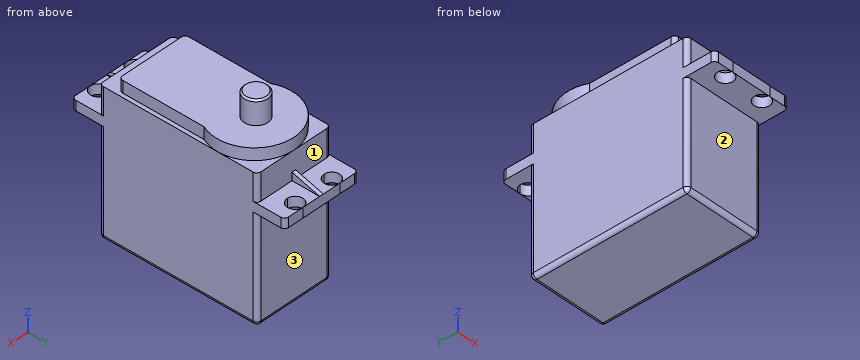
```python
from build123d import *

# Parameters (mm, degrees)
SKETCH_W        = 54
SKETCH_H        = 36
PAD_DEPTH       = 20
SKETCH001_W     = 7
SKETCH001_H     = 26.6
SKETCH001_H_2   = 6.9
POCKET_DEPTH    = 20.001
PAD001_DEPTH    = 3
SKETCH003_R     = 3
PAD002_DEPTH    = 45
SKETCH004_R     = 2
POCKET001_DEPTH = 2.5
PAD003_START    = -9.5
PAD003_DEPTH    = 1
CHAMFER_SIZE    = 0.4
FILLET_R        = 1
FILLET001_R     = 1
FILLET002_R     = 1


with BuildPart() as part:
    # Sketch → Pad (new body)
    with BuildSketch(Plane.YZ):
        with Locations((27, 18)):
            Rectangle(SKETCH_W, SKETCH_H)
    extrude(amount=PAD_DEPTH)

    # Sketch001 (on DatumPlane) → Pocket (cut, through all)
    with BuildSketch(Plane.YZ.offset(20)):
        with Locations((3.5, 13.3)):
            Rectangle(SKETCH001_W, SKETCH001_H)
        with Locations((50.5, 13.3)):
            Rectangle(SKETCH001_W, SKETCH001_H)
        with Locations((3.5, 32.55)):
            Rectangle(SKETCH001_W, SKETCH001_H_2)
        with Locations((50.5, 32.55)):
            Rectangle(SKETCH001_W, SKETCH001_H_2)
    extrude(amount=-POCKET_DEPTH, mode=Mode.SUBTRACT)

    # Sketch002 (on DatumPlane) → Pad001 (join)
    with BuildSketch(Plane(origin=(0, 0, 36), x_dir=(0, -1, 0), z_dir=(0, 0, 1))):
        with BuildLine():
            Line((-11, 19), (-32.641101, 19))
            ThreePointArc((-32.641101, 19), (-47, 10), (-32.641101, 1))
            Line((-32.641101, 1), (-11, 1))
            Line((-11, 1), (-11, 19))
        make_face()
    extrude(amount=PAD001_DEPTH)

    # Sketch003 → Pad002 (join)
    with BuildSketch(Plane.XY):
        with Locations((10, 37.4)):
            Circle(SKETCH003_R)
    extrude(amount=PAD002_DEPTH)

    # Sketch004 (on Face7 of Pad002) → Pocket001 (cut)
    with BuildSketch(Plane(origin=(0, 0, 29.1), x_dir=(0, -1, 0), z_dir=(0, 0, 1))):
        with Locations((-52, 15)):
            Circle(SKETCH004_R)
        with Locations((-52, 5)):
            Circle(SKETCH004_R)
        with Locations((-2, 15)):
            Circle(SKETCH004_R)
        with Locations((-2, 5)):
            Circle(SKETCH004_R)
    extrude(amount=-POCKET001_DEPTH, mode=Mode.SUBTRACT)

    # Sketch005 (on DatumPlane) → Pad003 (join)
    with BuildSketch(Plane.YZ.offset(20).offset(PAD003_START)):
        Polygon((0, 29.1), (7, 31.1), (7, 29.1), align=None)
        Polygon((54, 29.1), (47, 29.1), (47, 31.1), align=None)
    extrude(amount=-PAD003_DEPTH)

    # Chamfer
    chamfer_edges = [part.edges().sort_by_distance(p)[0] for p in [
        (7, 37.4, 45),
    ]]
    chamfer(chamfer_edges, length=CHAMFER_SIZE)

    # Fillet
    fillet_edges = [part.edges().sort_by_distance(p)[0] for p in [
        (0, 47, 13.3),
        (20, 47, 13.3),
        (0, 27, 0),
        (10, 47, 0),
        (20, 27, 0),
        (10, 7, 0),
        (0, 7, 13.3),
        (20, 7, 13.3),
        (20, 7, 32.55),
        (0, 7, 32.55),
        (20, 47, 32.55),
        (0, 47, 32.55),
    ]]
    fillet(fillet_edges, radius=FILLET_R)

    # Fillet001
    fillet001_edges = [part.edges().sort_by_distance(p)[0] for p in [
        (0, 54, 27.85),
        (20, 54, 27.85),
        (0, 0, 27.85),
        (20, 0, 27.85),
    ]]
    fillet(fillet001_edges, radius=FILLET001_R)

    # Fillet002
    fillet002_edges = [part.edges().sort_by_distance(p)[0] for p in [
        (1, 11, 37.5),
        (19, 11, 37.5),
    ]]
    fillet(fillet002_edges, radius=FILLET002_R)


solid = part.part
```
The listing builds one solid part. Answer for the finished solid, in the listing's coordinates (mm). Face numbers are marked on the shaded views. A direction names the side the tool comes from. Coordinates: 2 decimals unless noted, no trailing zeros. Write each loop counter-clockwise with the first axis right and the second up, starting at its lowest first coordinate (ties: lowest second). Pieces come first, ordered by that corner, then holes. Notation, with made-up numbers: M 80,70 L 111,70 A5 cw 111,74 Z; hole C 70.25,-34.75 d9. An arc over 180 degrees is marked long. Use a Markdown table: item, result. Add a question column.
1. Section D-D (x = 4) is taken. Give the vertices of the cut face in (y, z).
2. Section C-C (z = 33.5) is taken. Give the vertices of the cut face in (x, y).
3. Straight lines are drawn through the part: line 1 along X through (y, z) = (2, 28.25); line 2 along Z through (x, y) = (3.75, 32.5); line 3 along Y through (x, z) = (5.5, 35.5). For each, find the intervals that lie inside material, in ascending order. Write a range as [from, to].
4. Section B-B (y = 52) is taken. Give the vertices of the cut face in (x, z).
5. Which of the six approach directions +Z, -Z, +X, -X, +Y, -Y give full straight-line access (tool end or side, diameter ignored) to the marked faces 1, 2 and 3?
6. Given P1, Ø6.5, axis at x = 5, y = 2.5, coming from the +Z side; P2, Ø1.5, axis at x = 18, y = 37, coming from the +Z side; P3, Ø1.5, axis at y = 23.5, z = 38, coming from the +X side, each flat-ended and moving along its own axis, determine where each tip first touches the part or whether it passes through.
7. Section A-A (x = 15.75) is taken. Give the vertices of the cut face in (y, z).
Data:
| question | item | result |
|---|---|---|
| 1 | outline | M 0,26.6 L 0.27,26.6 L 0.27,29.1 L 0,29.1 Z; M 3.73,26.6 L 7,26.6 L 7,1 A1 ccw 8,0 L 46,0 A1 ccw 47,1 L 47,26.6 L 50.27,26.6 L 50.27,29.1 L 47,29.1 L 47,36 L 45,36 L 45,39 L 11,39 L 11,36 L 7,36 L 7,29.1 L 3.73,29.1 Z; M 53.73,26.6 L 54,26.6 L 54,29.1 L 53.73,29.1 Z |
| 2 | outline | M 0,8 A1 ccw 1,7 L 19,7 A1 ccw 20,8 L 20,46 A1 ccw 19,47 L 1,47 A1 ccw 0,46 Z |
| 3 | line 1 | x = [0, 3], [7, 13], [17, 20] |
| 3 | line 2 | z = [0, 39] |
| 3 | line 3 | y = [7, 47] |
| 4 | outline | M 0,26.6 L 3,26.6 L 3,29.1 L 0,29.1 Z; M 7,26.6 L 13,26.6 L 13,29.1 L 10.5,29.1 L 10.5,29.67 L 9.5,29.67 L 9.5,29.1 L 7,29.1 Z; M 17,26.6 L 20,26.6 L 20,29.1 L 17,29.1 Z |
| 5 | face 1 | +Z, +Y |
| 5 | face 2 | -Z, +X, -X, -Y |
| 5 | face 3 | -Z, +X, -X, +Y |
| 6 | P1 | stops at z = 29.1 |
| 6 | P2 | stops at z = 39 |
| 6 | P3 | stops at x = 19 |
| 7 | outline | M 0,26.6 L 0.15,26.6 L 0.15,29.1 L 0,29.1 Z; M 3.85,26.6 L 7,26.6 L 7,1 A1 ccw 8,0 L 46,0 A1 ccw 47,1 L 47,26.6 L 50.15,26.6 L 50.15,29.1 L 47,29.1 L 47,36 L 45.18,36 L 45.18,39 L 11,39 L 11,36 L 7,36 L 7,29.1 L 3.85,29.1 Z; M 53.85,26.6 L 54,26.6 L 54,29.1 L 53.85,29.1 Z |
